Check sheet for the modelled part. Datum: model origin and axes. Units: mm. Face numbers are marked on the shaded views. Give positions to 0.01 mm unless a question says otherwise; leave off trailing zeros. Order: outer loops, then holes, each group sorted by start corner. A loop starts at its lowest first (then second) coordinate and runs counter-clockwise, first axis right, second up.
Autodesk Inventor part; units mm, degrees
ref_plane "YZ Plane" through (0, 0, 0) normal (1, 0, 0) x (0, 1, 0)
ref_plane "XZ Plane" through (0, 0, 0) normal (0, 1, 0) x (-1, 0, 0)
ref_plane "XY Plane" through (0, 0, 0) normal (0, 0, 1) x (1, 0, 0)
sketch "Sketch1" plane through (0, 0, 0) normal (0, 0, 1) x (1, 0, 0)
  line L0 (178.5, -113.5) -> (-178.5, -113.5)
  line L1 (-178.5, -113.5) -> (-178.5, 113.5)
  line L2 (-178.5, 113.5) -> (178.5, 113.5)
  line L3 (178.5, 113.5) -> (178.5, -113.5)
  line L4 (178.5, -113.5) -> (-178.5, 113.5) construction
  line L5 (-178.5, -113.5) -> (178.5, 113.5) construction
  point P0 (0, 0)
  dimension "d0" = 357
  dimension "d1" = 227
extrude "Extrusion1" add sketch "Sketch1" along normal blind 5
sketch "Sketch2" plane through (0, 0, 5) normal (0, 0, 1) x (1, 0, 0)
  line L0 (37.5, -37.5) -> (-37.5, -37.5) construction
  line L1 (-37.5, -37.5) -> (-37.5, 37.5) construction
  line L2 (-37.5, 37.5) -> (37.5, 37.5) construction
  line L3 (37.5, 37.5) -> (37.5, -37.5) construction
  line L4 (37.5, -37.5) -> (-37.5, 37.5) construction
  line L5 (-37.5, -37.5) -> (37.5, 37.5) construction
  point P0 (0, 0)
  dimension "d4" = 75
  dimension "d5" = 75
hole "Hole1" at (-37.5, 37.5, 5) at (37.5, 37.5, 5) at (37.5, -37.5, 5) at (-37.5, -37.5, 5) direction (0, 0, -1) diameter 3 depth 3
fillet "Fillet1" radius 2 4 edges at (-178.5, 0, 0) (-178.5, 0, 5) (178.5, 0, 5) (178.5, 0, 0)
sketch "Sketch3" plane through (0, 0, 0) normal (0, 0, -1) x (-1, 0, 0)
  line L0 (168.1886, -102.5002) -> (-168.1886, -102.5002)
  line L1 (-168.1886, -102.5002) -> (-168.1886, 102.5002)
  line L2 (-168.1886, 102.5002) -> (168.1886, 102.5002)
  line L3 (168.1886, 102.5002) -> (168.1886, -102.5002)
  line L4 (168.1886, -102.5002) -> (-168.1886, 102.5002) construction
  line L5 (-168.1886, -102.5002) -> (168.1886, 102.5002) construction
  point P0 (0, 0)
extrude "Extrusion2" cut sketch "Sketch3" against normal blind 1
properties part number "Monitor"
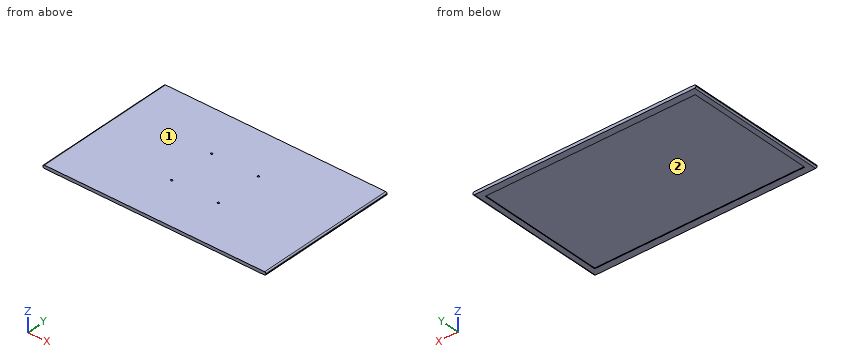
1) Section check A-A, the plane x = -143.5. Record the cut outline in (y, z).
Recorded:
outline: (-113.5, 0) - (-102.5, 0) - (-102.5, 1) - (102.5, 1) - (102.5, 0) - (113.5, 0) - (113.5, 5) - (-113.5, 5) - close
2) Material ranges on L1, parallel to Y at x = -37.5, z = 2.65; L2, parallel to X at y = 37.5, z = 3.5; L3, parallel to X at y = 37.5, z = 4.3, recorded low to high.
Recorded:
L1: y = -113.5 to -39, -36 to 36, 39 to 113.5
L2: x = -178.44 to -39, -36 to 36, 39 to 178.44
L3: x = -178.02 to -39, -36 to 36, 39 to 178.02
3) Section check B-B, the plane y = -55.5. Record the cut outline in (x, z).
Recorded:
outline: (-178.5, 2) arc R2 ccw to (-176.5, 0) - (-168.19, 0) - (-168.19, 1) - (168.19, 1) - (168.19, 0) - (176.5, 0) arc R2 ccw to (178.5, 2) - (178.5, 3) arc R2 ccw to (176.5, 5) - (-176.5, 5) arc R2 ccw to (-178.5, 3) - close
4) Depth check by flat-ended pin: pin 1 Ø1.1 at (y, z) = (44.5, 0.5) entering from -X; pin 2 Ø1.5 at (x, y) = (38, -37) entering from +Z; pin 3 Ø2.5 at (x, y) = (-37.5, 37.5) entering from -Z. Enter the tip coordinate at first touch or a pass-through.
Recorded:
pin 1: stops at x = -178.26
pin 2: stops at z = 2
pin 3: stops at z = 1
5) Draft check along X on the marked faces 1 and 2. Enter one of: +X half, -X half, draft (parallel to the pull), parting line (faces both ways), or undercut.
Recorded:
face 1: draft
face 2: undercut
